Model file for the job. Use its own axes, mm. A direction names the side the tool comes from. Coordinates: 2 decimals unless noted, no trailing zeros. Loops run counter-clockwise (first coordinate to the right, second up) from the corner with the lowest first, then second, coordinate; pieces in that order, holes last.
from build123d import *

# Parameters (mm, degrees)
BOSS_EXTRUDE2_DEPTH     = 25.4
SKETCH5_W               = 15.24
SKETCH5_H               = 25.4
BOSS_EXTRUDE3_DEPTH     = 12.7
SKETCH7_W               = 5.08
SKETCH7_H               = 25.4
CUT_EXTRUDE1_DEPTH      = 11.43
SKETCH8_R               = 3.175
CUT_EXTRUDE2_DEPTH      = 17.018
SKETCH9_R               = 2.54
CUT_EXTRUDE3_DEPTH      = 105.993449126
SKETCH10_W              = 5.08
SKETCH10_H              = 9.050505722
BOSS_EXTRUDE4_DEPTH     = 1.27
CHAMFER1_SIZE           = 1.27
CUT_EXTRUDE4_DEPTH      = 2.54
CUT_EXTRUDE4_DEPTH_BACK = 2.54
SKETCH12_W              = 2.770836572
SKETCH12_H              = 0.635
CUT_EXTRUDE5_DEPTH      = 51.805574613


with BuildPart() as part:
    # Sketch1 → Boss-Extrude2 (new body)
    with BuildSketch(Plane.XY):
        with BuildLine():
            Line((-93.89579229, 25.057477651), (-78.65579229, 25.057477651))
            ThreePointArc((-78.65579229, 25.057477651), (-86.27579229, 2.197477651), (-93.89579229, 25.057477651))
        make_face()
    extrude(amount=BOSS_EXTRUDE2_DEPTH)

    # Sketch5 → Boss-Extrude3 (add)
    with BuildSketch(Plane(origin=(0, 25.057477651, 0), x_dir=(1, 0, 0), z_dir=(0, 1, 0))):
        with Locations((-86.27579229, -12.7)):
            Rectangle(SKETCH5_W, SKETCH5_H)
    extrude(amount=BOSS_EXTRUDE3_DEPTH)

    # Sketch7 → Cut-Extrude1 (cut)
    with BuildSketch(Plane(origin=(0, 37.757477651, 0), x_dir=(1, 0, 0), z_dir=(0, 1, 0))):
        with Locations((-86.27579229, -12.7)):
            Rectangle(SKETCH7_W, SKETCH7_H)
    extrude(amount=-CUT_EXTRUDE1_DEPTH, mode=Mode.SUBTRACT)

    # Sketch8 → Cut-Extrude2 (cut)
    with BuildSketch(Plane(origin=(-78.65579229, 0, 0), x_dir=(0, 0, -1), z_dir=(1, 0, 0))):
        with Locations((-12.7, 32.677477651)):
            Circle(SKETCH8_R)
        with BuildLine():
            Line((-12.7, 37.757477651), (0, 37.757477651))
            Line((0, 37.757477651), (0, 25.057477651))
            Line((0, 25.057477651), (-8.750796536, 35.872816757))
            ThreePointArc((-8.750796536, 35.872816757), (-10.512069775, 37.262165353), (-12.7, 37.757477651))
        make_face()
    extrude(amount=-CUT_EXTRUDE2_DEPTH, mode=Mode.SUBTRACT)

    # Sketch9 → Cut-Extrude3 (cut, through all)
    with BuildSketch(Plane(origin=(0, 26.327477651, 0), x_dir=(1, 0, 0), z_dir=(0, 1, 0))):
        with Locations(Location((-86.27579229, -12.7, 0), (0, 0, 270))):
            Circle(SKETCH9_R)
    extrude(amount=-CUT_EXTRUDE3_DEPTH, mode=Mode.SUBTRACT)

    # Sketch10 → Boss-Extrude4 (add)
    with BuildSketch(Plane(origin=(0, 37.757477651, 0), x_dir=(1, 0, 0), z_dir=(0, 1, 0))):
        with Locations((-91.35579229, -20.874747139)):
            Rectangle(SKETCH10_W, SKETCH10_H)
        with Locations((-81.19579229, -20.874747139)):
            Rectangle(SKETCH10_W, SKETCH10_H)
    extrude(amount=BOSS_EXTRUDE4_DEPTH)

    # Chamfer1
    chamfer1_edges = [part.edges().sort_by_distance(p)[0] for p in [
        (-81.19579229, 39.027477651, 16.349494278),
        (-91.35579229, 39.027477651, 16.349494278),
    ]]
    chamfer(chamfer1_edges, length=CHAMFER1_SIZE - 0.0001)  # a hair under: the kernel refuses the full size

    # Sketch11 → Cut-Extrude4 (cut, two sides: drawn at the far end of the back side and taken through both)
    with BuildSketch(Plane.XY.offset(12.7).offset(-CUT_EXTRUDE4_DEPTH_BACK)):
        with BuildLine():
            Line((-88.81579229, 26.327477651), (-93.000878218, 4.124213556))
            ThreePointArc((-93.000878218, 4.124213556), (-86.27579229, 2.197477651), (-79.550706362, 4.124213556))
            Line((-79.550706362, 4.124213556), (-83.73579229, 26.327477651))
            Line((-83.73579229, 26.327477651), (-88.81579229, 26.327477651))
        make_face()
    extrude(amount=CUT_EXTRUDE4_DEPTH + CUT_EXTRUDE4_DEPTH_BACK, mode=Mode.SUBTRACT)

    # Sketch12 → Cut-Extrude5 (cut, through all)
    with BuildSketch(Plane(origin=(-78.65579229, 0, 0), x_dir=(0, 0, -1), z_dir=(1, 0, 0))):
        with Locations((-12.7, 26.009977651)):
            Rectangle(SKETCH12_W, SKETCH12_H)
        with Locations((-12.7, 27.279977651)):
            Rectangle(SKETCH12_W, SKETCH12_H)
    extrude(amount=-CUT_EXTRUDE5_DEPTH, mode=Mode.SUBTRACT)


solid = part.part
Q1. Slice it at A-A (z = 14.5). List the corners of the cut face in (x, y), and give its area (3 significant figures).
Answers:
outline: (-93.9, 25.06) arc R12.7 ccw to (-93, 4.12) - (-88.82, 26.33) - (-88.82, 30.06) - (-93.9, 30.06) - close; (-93.9, 35.29) - (-88.82, 35.29) - (-88.82, 37.76) - (-93.9, 37.76) - close; (-83.74, 26.33) - (-79.55, 4.12) arc R12.7 ccw to (-78.66, 25.06) - (-78.66, 30.06) - (-83.74, 30.06) - close; (-83.74, 35.29) - (-78.66, 35.29) - (-78.66, 37.76) - (-83.74, 37.76) - close
area: 339 mm2
Q2. Slice it at D-D (x = -85.5). List the corners of the cut face in (y, z).
Answers:
outline: (2.22, 0) - (25.06, 0) - (26.33, 1.03) - (26.33, 10.16) - (2.22, 10.16) - close; (2.22, 15.24) - (26.33, 15.24) - (26.33, 25.4) - (2.22, 25.4) - close
Q3. Slice it at C-C (y = 24). List the corners of the cut face in (x, z).
Answers:
outline: (-95.13, 0) - (-77.42, 0) - (-77.42, 25.4) - (-95.13, 25.4) - close; hole (-89.25, 10.16) - (-83.3, 10.16) - (-83.3, 15.24) - (-89.25, 15.24) - close
Q4. Which spindle directions (+Z, -Z, +X, -X, +Y, -Y) get a long thin tool onto all of the face, cutting with end or side? Do faces 1 (the flat face through (-83, 30, 4)), 2 (the flat face through (-81, 27.597, 13)), 3 (the flat face through (-86, 12, 15.24)). Say none if no direction does.
Answers:
face 1: -Z, +X, -X, +Y
face 2: +X, -X
face 3: -Y
Q5. Flat gauge pins, fed straight in: P1, Ø1.5, axis at y = 32.5, z = 4.5, coming from the -X side; P2, Ø14, axis at y = 33.5, z = 17, coming from the +X side; P3, Ø4, axis at x = -85, z = 4.5, coming from the +Y side; P4, Ø6, axis at x = -94.5, z = 17, coming from the -Y side. Where does each tip first touch, or does it go through?
Answers:
P1: passes through
P2: stops at x = -78.66
P3: stops at y = 32.53
P4: stops at y = 3.32
Q6. Drill centre lines: line 1 (Z direction, x = -90.5, y = 5); line 2 (X direction, y = 30, z = 23); line 3 (X direction, y = 7.5, z = 15). Where is each one in solid material? Low to high.
Answers:
line 1: z = 0 to 10.16, 15.24 to 25.4
line 2: x = -93.9 to -88.82, -83.74 to -78.66
line 3: x = -96.6 to -92.36, -80.19 to -75.95
Q7. Mould opens along Z. For faces 4 (the flat face through (-91, 39.027, 21)), 5 (the cylindrical face through (-91.32, 35.355, 10.993)), 6 (the flat face through (-86, 20, 25.4)) say: +Z half, -Z half, draft (parallel to the pull), parting line (faces both ways), or undercut.
Answers:
face 4: draft
face 5: undercut
face 6: +Z half
Q8. Slice it at B-B (x = -80.75). Count the separate pieces of the cut face and the enclosed holes in it, and give its area (3 significant figures).
Answers:
separate pieces: 1
enclosed holes: 3
area: 745 mm2
